from build123d import *

# Parameters (mm, degrees)
F3_DEPTH = 140
F5_D     = 24
F5_DEPTH = 100
F5_TIP   = 7.2103274283


with BuildPart() as f1:
    # F0 (on Front) → F1 (revolve)
    with BuildSketch(Plane.XZ):
        Polygon((-1.5155260398, 80.1515013238), (-1.6437353146, 64.1515013238), (-171.6437353146, 65.5137248684), (-171.6437353146, -1.8484986762), (-116.1690213024, -1.8484986762), (-60.6943072902, -1.8484986762), (29.2721830071, -1.8484986762), (68.3562646854, -1.8484986762), (68.3562646856, 79.3194004249), (68.3562646856, 146.1515013238), (-56.7185516386, 146.1515013238), align=None)
        with BuildLine():
            Line((-60.6943072902, -1.8484986762), (-116.1690213024, -1.8484986762))
            Line((-116.1690213024, -1.8484986762), (-130.0498999893, -21.8484986762))
            Line((-130.0498999893, -21.8484986762), (-130.0498999893, -61.8484986762))
            Line((-130.0498999893, -61.8484986762), (22.9833192886, -61.8484986762))
            ThreePointArc((22.9833192886, -61.8484986762), (3.9159803894, -29.5203853555), (29.2721830071, -1.8484986762))
            Line((29.2721830071, -1.8484986762), (-60.6943072902, -1.8484986762))
        make_face()
        Polygon((22.9833192886, -61.8484986762), (-130.0498999893, -61.8484986762), (-191.2617840111, -61.8484986762), (-191.1197163402, -75.8484986762), (45.0953505933, -75.8484986762), (83.0453708768, -50.2909868956), (213.9352560043, -50.2909868956), (213.9352560043, -36.6648137569), (80.4508551955, -36.6648137569), (41.0931288958, -61.8484986762), align=None)
    revolve(axis=Axis((-18.4481963515, 0, -181.8484986762), (1, 0, 0)))

    # F2 (on face) → F3 (cut)
    with BuildSketch(Plane(origin=(-130.0498999893, 0, 0), x_dir=(0, -1, 0), z_dir=(-1, 0, 0))):
        with BuildLine():
            Line((31.2392264938, -65.9860339689), (45.9312041985, -28.6587765722))
            ThreePointArc((45.9312041985, -28.6587765722), (0, -21.921119915), (-45.9312041985, -28.6587765722))
            Line((-45.9312041985, -28.6587765722), (-31.2392264938, -65.9860339689))
            ThreePointArc((-31.2392264938, -65.9860339689), (0, -61.8484986762), (31.2392264938, -65.9860339689))
        make_face()
        with BuildLine():
            Line((155.63179304, -218.665770066), (115.9594510286, -212.7257672917))
            ThreePointArc((115.9594510286, -212.7257672917), (103.9230484541, -241.8484986762), (84.7202245348, -266.8336947681))
            Line((84.7202245348, -266.8336947681), (109.7005888416, -298.2209493906))
            ThreePointArc((109.7005888416, -298.2209493906), (138.5011727679, -261.8121880569), (155.63179304, -218.665770066))
        make_face()
        with BuildLine():
            Line((109.7005888416, -65.4760479619), (84.7202245348, -96.8633025843))
            ThreePointArc((84.7202245348, -96.8633025843), (103.9230484541, -121.8484986762), (115.9594510286, -150.9712300607))
            Line((115.9594510286, -150.9712300607), (155.63179304, -145.0312272865))
            ThreePointArc((155.63179304, -145.0312272865), (138.5011727679, -101.8848092956), (109.7005888416, -65.4760479619))
        make_face()
        with BuildLine():
            ThreePointArc((31.2392264938, -297.7109633836), (0, -301.8484986762), (-31.2392264938, -297.7109633836))
            Line((-31.2392264938, -297.7109633836), (-45.9312041985, -335.0382207803))
            ThreePointArc((-45.9312041985, -335.0382207803), (0, -341.7758774375), (45.9312041985, -335.0382207803))
            Line((45.9312041985, -335.0382207803), (31.2392264938, -297.7109633836))
        make_face()
        with BuildLine():
            ThreePointArc((-84.7202245348, -266.8336947681), (-103.9230484541, -241.8484986762), (-115.9594510286, -212.7257672917))
            Line((-115.9594510286, -212.7257672917), (-155.63179304, -218.665770066))
            ThreePointArc((-155.63179304, -218.665770066), (-138.5011727679, -261.8121880569), (-109.7005888416, -298.2209493906))
            Line((-109.7005888416, -298.2209493906), (-84.7202245348, -266.8336947681))
        make_face()
        with BuildLine():
            ThreePointArc((-115.9594510286, -150.9712300607), (-103.9230484541, -121.8484986762), (-84.7202245348, -96.8633025843))
            Line((-84.7202245348, -96.8633025843), (-109.7005888416, -65.4760479619))
            ThreePointArc((-109.7005888416, -65.4760479619), (-138.5011727679, -101.8848092956), (-155.63179304, -145.0312272865))
            Line((-155.63179304, -145.0312272865), (-115.9594510286, -150.9712300607))
        make_face()
    extrude(amount=-F3_DEPTH, mode=Mode.SUBTRACT)

    # F5
    with Locations(Plane(origin=(-171.6437353146, 0, 0), x_dir=(0, -1, 0), z_dir=(-1, 0, 0))):
        with Locations((-115, 17.3373441942), (0, 48.1515013238), (115, 17.3373441942), (199.1858428704, -66.8484986762), (230, -181.8484986762), (-199.1858428704, -66.8484986762), (-230, -181.8484986762), (-199.1858428704, -296.8484986762), (-115, -381.0343415467), (0, -411.8484986762), (115, -381.0343415467), (199.1858428704, -296.8484986762)):
            Hole(F5_D / 2, depth=F5_DEPTH)
            with Locations((0, 0, -(F5_DEPTH + F5_TIP / 2))):  # 118° drill point
                Cone(0, F5_D / 2, F5_TIP, mode=Mode.SUBTRACT)


solid = f1.part
The listing builds one solid part. Answer for the finished solid, in the listing's coordinates (mm). A direction names the side the tool comes from. Round coordinates to 2 decimals unless told otherwise and drop trailing zeros. Order: outer loops, then holes, each group sorted by start corner. A loop starts at its lowest first (then second) coordinate and runs counter-clockwise, first axis right, second up. Notation, with made-up numbers: (-7.75, -0.5) - (35.25, -0.5) arc R32 ccw to (35.25, 31.5) - close; hole circle Ø7 at (42.5, 16.25). An arc over 180 degrees is marked (long way). Write item = value, one per line. Start each with the question number.
1) Section B-B, the plane x = 58 is taken. Write down the section's boundary in (y, z), plus the area to 3 significant figures.
2) Section A-A, the plane x = -152 is taken. Count the separate pieces of the cut face and the enclosed holes in it, plus the area to 3 significant figures.
3) Given pin 1 (19 mm diameter, centred on y = -115, z = -381.03, fed in from -X); pin 2 (5 mm diameter, centred on x = -148, y = 162.5, fed in from -Z); pin 3 (3 mm diameter, centred on x = -3, z = -328, fed in from +Y), each flat-ended and moving along its own axis, determine where each tip first touches the part or whether it passes through.
4) Straight lines are drawn through the part: L1, parallel to Z at x = -155.5, y = -19.5; L2, parallel to Z at x = -135, y = 0; L3, parallel to Z at x = -128, y = 204.5. For each, find the intervals that lie inside material, in ascending order.
5) For faces 1 (the cylindrical face through (31.911, -81.102, -270.293)), 2 (the conical face through (47.47, -32.32, -79.22)), 3 (the cylindrical face through (-120.94, 103.01, 17.86)), determine the directions among +Z, -Z, +X, -X, +Y, -Y from which every point of the face is accessible in a straight line to the end or side of a thin tool.
6) Section C-C, the plane x = 153.5 is taken. Write down the section's boundary in (y, z), plus the area to 3 significant figures.
Results list:
q1.outline = circle Ø656 at (0, -181.85); circle Ø261.64 at (0, -181.85); hole circle Ø360 at (0, -181.85); hole circle Ø229.38 at (0, -181.85)
q1.area = 249,000 mm^2
q2.separate_pieces = 2
q2.enclosed_holes = 14
q2.area = 94,700 mm^2
q3.pin_1 = -70.14
q3.pin_2 = -370.25
q3.pin_3 = 294.38
q4.L1 = -428.31 to -360.79, -300.25 to -286.04, -77.66 to -63.44, -2.91 to 64.61
q4.L2 = -428.92 to -423.85, -399.85 to -361.85, -301.85 to -287.85, -75.85 to -61.85, -1.85 to 36.15, 60.15 to 65.22
q4.L3 = -320.39 to -307.61, -286.09 to -77.61, -56.09 to -43.3
q5.face_1 = none
q5.face_2 = +X
q5.face_3 = -X
q6.outline = circle Ø290.37 at (0, -181.85); hole circle Ø263.12 at (0, -181.85)
q6.area = 11,800 mm^2
